Design review of the part shown in the three views and the two pictorial views. Dimensions are in mm from the part's minimum x, y and z. Coordinates: 2 decimals unless noted, no trailing zeros. Write each loop counter-clockwise with the first axis right and the second up, starting at its lowest first coordinate (ties: lowest second). Pieces come first, ordered by that corner, then holes.
Q1. For pin 1 Ø1 at (x, z) = (7, 2) entering from +Y; pin 2 Ø1.5 at (y, z) = (8.5, 3) entering from +X, all flat-tipped, find the tip position at first contact; note any pin that passes through.
Q2. For L1, parallel to X at y = 4.25, z = 3.05; L2, parallel to X at y = 8.5, z = 3; L3, parallel to Y at x = 2.25, z = 3.45, list the stretches that pass through material, from the lowest coordinate up.
Q3. Take a section at D-D, the plane z = 2.7. Write out the cut boundary in (x, y).
Q4. Take a section at C-C, the plane y = 8.8. Write out the cut boundary in (x, z).
Q5. Take a section at A-A, the plane x = 6. Write out the cut boundary in (y, z).
Q6. The part is to be moulded in two halves that separate along X. For the marked faces 1, 2 and 3, say which applies: released by +X, released by -X, zero draft, split by the parting line, or undercut.
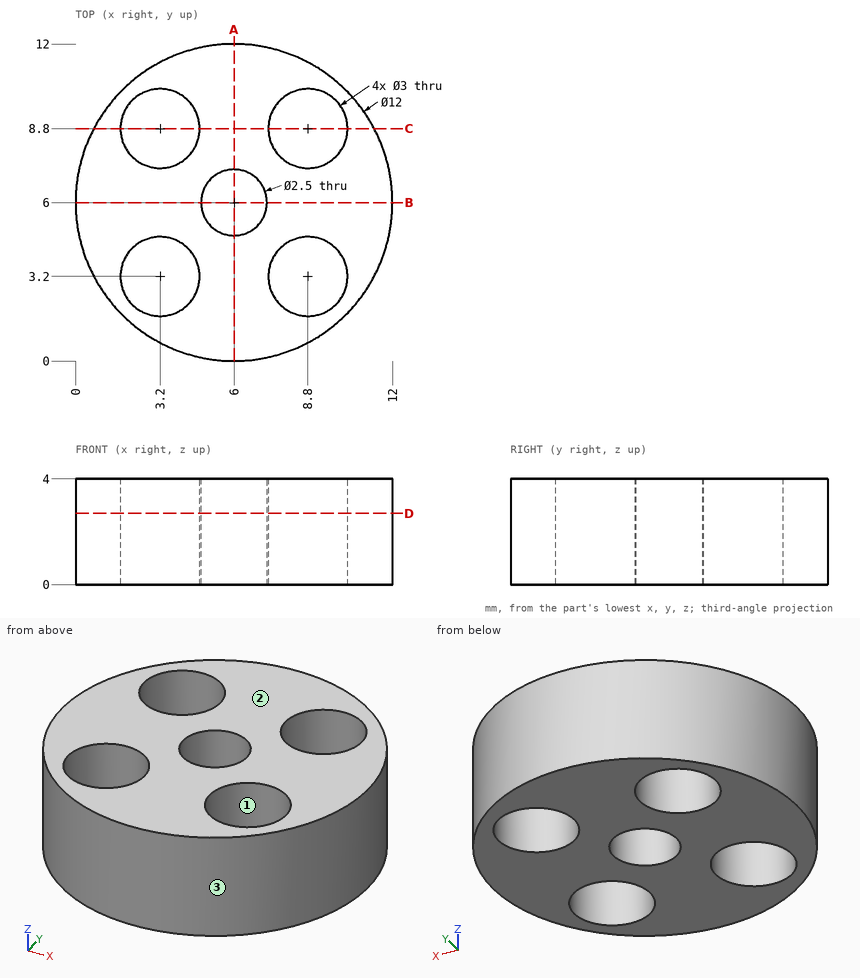
Responses:
1. pin 1: stops at y = 11.98
1. pin 2: stops at x = 11.74
2. L1: x = 0.26 to 2.13, 4.27 to 7.73, 9.87 to 11.74
2. L2: x = 0.55 to 1.73, 4.67 to 7.33, 10.27 to 11.45
2. L3: y = 1.32 to 2.04, 4.36 to 7.64, 9.96 to 10.68
3. outline: circle Ø12 at (6, 6); hole circle Ø3 at (3.2, 3.2); hole circle Ø3 at (3.2, 8.8); hole circle Ø2.5 at (6, 6); hole circle Ø3 at (8.8, 3.2); hole circle Ø3 at (8.8, 8.8)
4. outline: (0.69, 0) - (1.7, 0) - (1.7, 4) - (0.69, 4) - close; (4.7, 0) - (7.3, 0) - (7.3, 4) - (4.7, 4) - close; (10.3, 0) - (11.31, 0) - (11.31, 4) - (10.3, 4) - close
5. outline: (0, 0) - (4.75, 0) - (4.75, 4) - (0, 4) - close; (7.25, 0) - (12, 0) - (12, 4) - (7.25, 4) - close
6. face 1: undercut
6. face 2: zero draft
6. face 3: split by the parting line
